from build123d import *

# Parameters (mm, degrees)
BASE_FLANGE1_DEPTH = 40
SKETCH7_R          = 4
CUT_EXTRUDE1_DEPTH = 2
CUT_EXTRUDE2_DEPTH = 2


# Sheet-metal steps are written as plain solids
with BuildPart() as part:
    # Sketch1 → Base-Flange1 (new body)
    with BuildSketch(Plane(origin=(0, 0, 0), x_dir=(0, 0, -1), z_dir=(1, 0, 0))):
        with BuildLine():
            Line((0, 0), (399.171572875, 0))
            ThreePointArc((399.171572875, 0), (399.93693974, 0.152240935), (400.585786438, 0.585786438))
            Line((400.585786438, 0.585786438), (449.497474683, 49.497474683))
            Line((449.497474683, 49.497474683), (450.911688245, 48.083261121))
            Line((450.911688245, 48.083261121), (402, -0.828427125))
            ThreePointArc((402, -0.828427125), (400.702306605, -1.69551813), (399.171572875, -2))
            Line((399.171572875, -2), (0, -2))
            Line((0, -2), (0, 0))
        make_face()
    extrude(amount=BASE_FLANGE1_DEPTH)

    # Sketch7 → Cut-Extrude1 (cut)
    with BuildSketch(Plane(origin=(0, -200, -200), x_dir=(1, 0, 0), z_dir=(0, 0.7071067811865456, 0.7071067811865496))):
        with Locations(Location((20, 317.842712475, 0), (0, 0, 270))):
            Circle(SKETCH7_R)
    extrude(amount=-CUT_EXTRUDE1_DEPTH, mode=Mode.SUBTRACT)

    # Sketch8 → Cut-Extrude2 (cut)
    with BuildSketch(Plane(origin=(0, 0, 0), x_dir=(1, 0, 0), z_dir=(0, 1, 0))):
        with BuildLine():
            Line((24, 50), (24, 250))
            ThreePointArc((24, 250), (20, 254), (16, 250))
            Line((16, 250), (16, 50))
            ThreePointArc((16, 50), (20, 46), (24, 50))
        make_face()
    extrude(amount=-CUT_EXTRUDE2_DEPTH, mode=Mode.SUBTRACT)


solid = part.part
Geometry: final body of the model. Coordinates: model frame, mm. A direction names the side the tool comes from. Round coordinates to 2 decimals unless told otherwise and drop trailing zeros. Order: outer loops, then holes, each group sorted by start corner. A loop starts at its lowest first (then second) coordinate and runs counter-clockwise, first axis right, second up.
Q1. Section C-C, the plane z = -313.5. Output: boundary loops of the cut face in (x, y).
Result sheet:
outline: (0, -2) - (40, -2) - (40, 0) - (0, 0) - close
Q2. Material intervals for probe 1 along Y at (x, z) = (14, -227); probe 2 along Z at (x, y) = (9, 31.5); probe 3 along Z at (x, y) = (26, 13), sorted ascending.
Result sheet:
probe 1: y = -2 to 0
probe 2: z = -434.33 to -431.5
probe 3: z = -415.83 to -413
Q3. Section D-D, the plane y = 5.5. Output: boundary loops of the cut face in (x, z).
Result sheet:
outline: (0, -408.33) - (40, -408.33) - (40, -405.5) - (0, -405.5) - close
Q4. Access query for faces 1 (the face through (40, -1, -227)), 2 (the face through (15, 0, -197)). Directions: +Z, -Z, +X, -X, +Y, -Y. A direction counts if a zero-diameter tool reaches every point of the face in a straight line with its end or side. Return the directions, or none.
Result sheet:
face 1: +Z, -Z, +X, +Y, -Y
face 2: +Z, +X, -X, +Y
Q5. Section A-A, the plane z = -159. Output: boundary loops of the cut face in (x, y), and give its area (3 significant figures).
Result sheet:
outline: (0, -2) - (16, -2) - (16, 0) - (0, 0) - close; (24, -2) - (40, -2) - (40, 0) - (24, 0) - close
area: 64.0 mm2
Q6. Pin query (flat end, axial travel): pin 1 (8 mm diameter, centred on x = 11.5, z = -113.5, fed in from +Y); pin 2 (1 mm diameter, centred on x = 30.5, y = 40, fed in from -Z); pin 3 (5 mm diameter, centred on x = 34.5, y = 33, fed in from -Z). Return the tip coordinate at first contact, or that it passes through.
Result sheet:
pin 1: stops at y = 0
pin 2: stops at z = -443.33
pin 3: stops at z = -438.33
Q7. Section B-B, the plane x = 28. Output: boundary loops of the cut face in (y, z), and give its area (3 significant figures).
Result sheet:
outline: (-2, -399.17) arc R4 ccw to (-0.83, -402) - (48.08, -450.91) - (49.5, -449.5) - (0.59, -400.59) arc R2 cw to (0, -399.17) - (0, 0) - (-2, 0) - close
area: 941 mm2
